from build123d import *

# Parameters (mm, degrees)
F1_DEPTH = 2.5
F3_DEPTH = 6
F5_DEPTH = 100


with BuildPart() as f1:
    # F0 (on Top) → F1 (new body)
    with BuildSketch(Plane.XY):
        with BuildLine():
            Line((-79.815194, 68.501485), (-25, 13.686292))
            Line((-25, 13.686292), (-25, -13.686292))
            Line((-25, -13.686292), (-79.815194, -68.501485))
            ThreePointArc((-79.815194, -68.501485), (-88.131728, -88.131728), (-68.501485, -79.815194))
            Line((-68.501485, -79.815194), (-28.686292, -40))
            Line((-28.686292, -40), (28.686292, -40))
            Line((28.686292, -40), (68.501485, -79.815194))
            ThreePointArc((68.501485, -79.815194), (88.131728, -88.131728), (79.815194, -68.501485))
            Line((79.815194, -68.501485), (25, -13.686292))
            Line((25, -13.686292), (25, 13.686292))
            Line((25, 13.686292), (79.815194, 68.501485))
            ThreePointArc((79.815194, 68.501485), (88.131728, 88.131728), (68.501485, 79.815194))
            Line((68.501485, 79.815194), (28.686292, 40))
            Line((28.686292, 40), (-28.686292, 40))
            Line((-28.686292, 40), (-68.501485, 79.815194))
            ThreePointArc((-68.501485, 79.815194), (-88.131728, 88.131728), (-79.815194, 68.501485))
        make_face()
    extrude(amount=F1_DEPTH)

    # F2 (on Top) → F3 (join)
    with BuildSketch(Plane.XY):
        Polygon((-29.928932, -37), (-71.603911, -78.674978), (-68.501485, -79.815194), (-28.686292, -40), (28.686292, -40), (68.501485, -79.815194), (71.603911, -78.674978), (29.928932, -37), align=None)
        Polygon((-78.674978, -71.603911), (-22, -14.928932), (-22, 14.928932), (-78.674978, 71.603911), (-79.815194, 68.501485), (-25, 13.686292), (-25, -13.686292), (-79.815194, -68.501485), align=None)
        Polygon((22, 14.928932), (22, -14.928932), (78.674978, -71.603911), (79.815194, -68.501485), (25, -13.686292), (25, 13.686292), (79.815194, 68.501485), (78.674978, 71.603911), align=None)
        Polygon((29.928932, 37), (71.603911, 78.674978), (68.501485, 79.815194), (28.686292, 40), (-28.686292, 40), (-68.501485, 79.815194), (-71.603911, 78.674978), (-29.928932, 37), align=None)
    extrude(amount=-F3_DEPTH)

    # F4 (on Front) → F5 (cut, symmetric)
    with BuildSketch(Plane.XZ):
        Polygon((-28.709985, -15.796961), (-28.709985, -6.029143), (-91.463856, 0), (-91.463856, -15.796961), align=None)
        Polygon((28.709985, -6.029143), (28.709985, -15.796961), (91.463856, -15.796961), (91.463856, 0), align=None)
    extrude(amount=F5_DEPTH, both=True, mode=Mode.SUBTRACT)


solid = f1.part
Verification items for the finished model (mm, model axes). A direction names the side the tool comes from. Round coordinates to 2 decimals unless told otherwise and drop trailing zeros. Loops run counter-clockwise (first coordinate to the right, second up) from the corner with the lowest first, then second, coordinate; pieces in that order, holes last. Notation, with made-up numbers: (28, -33.75) - (72, -33.75) arc R20 cw to (72, -8.75) - close; hole circle Ø10 at (16.25, 28.5). An arc over 180 degrees is marked (long way). Use one line per item in the form item = value.
1. Draft check along Y on faces 4 (the flat face through (-48.632, 58.507, -4.115)), 5 (the flat face through (48.873, 60.186, -0.746)), 6 (the flat face through (48.315, -59.629, -0.746)), 7 (the flat face through (46.43, -53.5, -2.26)). Enter one of: pulls with the +Y half, pulls with the -Y half, needs draft (parallel to the pull), parting line crosses it, or undercut.
A:
face_4 = needs draft
face_5 = pulls with the +Y half
face_6 = pulls with the -Y half
face_7 = undercut
2. Gauge pin test, flat ends, axial feed: pin 1 Ø12 at (x, y) = (71, -59.5) entering from -Z; pin 2 Ø5 at (x, z) = (-14.5, -2.5) entering from +Y; pin 3 Ø5 at (x, z) = (-0.5, -3) entering from -Y. Record the tip position at first contact, or that the pin passes through.
A:
pin_1 = -2.53
pin_2 = 40
pin_3 = -40
3. Section check B-B on z = -3.5. Give the number of separate pieces and of enclosed holes in the cut face, and give its area (3 significant figures).
A:
separate_pieces = 4
enclosed_holes = 0
area = 1,500 mm²
4. Section check C-C on y = -5.5. Record the cut outline in (x, z), and give its area (3 significant figures).
A:
outline = (-25, -6) - (-22, -6) - (-22, 0) - (22, 0) - (22, -6) - (25, -6) - (25, 2.5) - (-25, 2.5) - close
area = 161 mm²
5. Scan lines: probe 1 along Y at (x, z) = (2.5, -5); probe 2 along Z at (x, y) = (-47, 51); probe 3 along X at (y, z) = (63.5, 1.25). Record each from-to range of solid material in increasing order.
A:
probe_1 = -40 to -37, 37 to 40
probe_2 = 0 to 2.5
probe_3 = -74.81 to -52.19, 52.19 to 74.81
6. Access from +Z, -Z, +X, -X, +Y, -Y to the whole of each face (thin tool, end or side, straight path). Record for faces 1 (the flat face through (-25, 0, -2)), 2 (the flat face through (0, -37, -3)), 3 (the flat face through (25, 0, -2)).
A:
face_1 = +Z, -Z, -X
face_2 = -Z
face_3 = +Z, -Z, +X
7. Section check A-A on x = 33. Record the cut outline in (y, z), and give its area (3 significant figures).
A:
outline = (-44.31, -5.62) - (-40.07, -5.62) - (-40.07, 0) - (-25.93, 0) - (-25.93, -5.62) - (-21.69, -5.62) - (-21.69, 2.5) - (-44.31, 2.5) - close; (21.69, -5.62) - (25.93, -5.62) - (25.93, 0) - (40.07, 0) - (40.07, -5.62) - (44.31, -5.62) - (44.31, 2.5) - (21.69, 2.5) - close
area = 208 mm²
8. Section check D-D on x = -14. Record the cut outline in (y, z).
A:
outline = (-40, -6) - (-37, -6) - (-37, 0) - (37, 0) - (37, -6) - (40, -6) - (40, 2.5) - (-40, 2.5) - close
